Build history of the part. All positions in model axes, mm. Face numbers are marked on the shaded views. A direction names the side the tool comes from. Coordinates: 2 decimals unless noted, no trailing zeros. Order: outer loops, then holes, each group sorted by start corner. A loop starts at its lowest first (then second) coordinate and runs counter-clockwise, first axis right, second up. Notation, with made-up numbers: M 33.5,50 L 81.5,50 A22 cw 81.5,61 Z; hole C -27,50.5 d11. An arc over 180 degrees is marked long. Write item = value, one per line. Start each with the question number.
Q1. Band-saw the part on D-D on y = 1.3. Write the cut outline in (x, z), plus the area to 3 significant figures.
Q2. Pull direction X, two halves, no side cores. Call the marked faces 1, 2 and 3: released by +X, released by -X, zero draft, split by the parting line, or undercut.
Q3. Band-saw the part on C-C on y = 2.35. Write the cut outline in (x, z), plus the area to 3 significant figures.
Q4. Band-saw the part on B-B on z = 0. Write the cut outline in (x, y).
Q5. 3-axis set-ups, long thin cutter, end or side, ignore diameter. For the marked faces 4 and 5: which of +Z, -Z, +X, -X, +Y, -Y reach the whole face in a straight line?
Q6. Pin check, flat tips, straight feed: P1, Ø1.5, axis at x = -3.5, z = 1, coming from the -Y side; P2, Ø1.5, axis at y = 2.5, z = -2, coming from the +X side; P3, Ø1, axis at y = 3, z = 0, coming from the +X side. Stop position of each tip, or through.
Q7. Drill centre lines: probe 1 along X at (y, z) = (1.45, -0.25); probe 2 along X at (y, z) = (2.3, 0); probe 3 along Z at (x, y) = (1.75, 0.3). Where is each one in solid material? Low to high.
Q8. Band-saw the part on A-A on x = 0. Write the cut outline in (y, z), plus the area to 3 significant figures.
```python
from build123d import *

# Parameters (mm, degrees)
SKETCH2_R          = 0.5
CUT_EXTRUDE1_DEPTH = 8.329743599


with BuildPart() as part:
    # Sketch1 → Revolve1 (revolve)
    with BuildSketch(Plane.XY, mode=Mode.PRIVATE) as revolve1_sk:
        Polygon((0, 0), (3, 0), (2.5, 0.657540642), (3.702619215, 1.572023442), (3, 2.496024821), (4.5, 3.636638726), (0, 3.636638726), align=None)
    revolve(revolve1_sk.sketch.rotate(Axis((0, 3.636638726, 0), (0, -1, 0)), 90), axis=Axis((0, 3.636638726, 0), (0, -1, 0)))

    # Sketch2 → Cut-Extrude1 (cut, through all)
    with BuildSketch(Plane(origin=(0, 3.636638726, 0), x_dir=(1, 0, 0), z_dir=(0, 1, 0))):
        with Locations(Location((0, 0, 0), (0, 0, 270))):
            Circle(SKETCH2_R)
    extrude(amount=-CUT_EXTRUDE1_DEPTH, mode=Mode.SUBTRACT)


solid = part.part
```
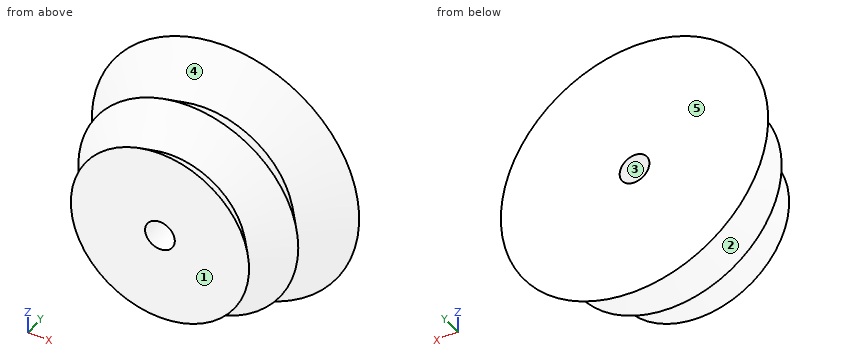
Recorded:
q1.outline = C 0,0 d6.69; hole C 0,0 d1
q1.area = 34.4 mm2
q2.face_1 = zero draft
q2.face_2 = split by the parting line
q2.face_3 = undercut
q3.outline = C 0,0 d6.22; hole C 0,0 d1
q3.area = 29.6 mm2
q4.outline = M -4.5,3.64 L -3,2.5 L -3.7,1.57 L -2.5,0.66 L -3,0 L -0.5,0 L -0.5,3.64 Z; M 0.5,0 L 3,0 L 2.5,0.66 L 3.7,1.57 L 3,2.5 L 4.5,3.64 L 0.5,3.64 Z
q5.face_4 = none
q5.face_5 = +Z, -Z, +X, -X, +Y
q6.P1 = 0
q6.P2 = 3.52
q6.P3 = 4.32
q7.probe_1 = -3.53 to -0.43, 0.43 to 3.53
q7.probe_2 = -3.15 to -0.5, 0.5 to 3.15
q7.probe_3 = -2.15 to 2.15
q8.outline = M 0,-3 L 0.66,-2.5 L 1.57,-3.7 L 2.5,-3 L 3.64,-4.5 L 3.64,-0.5 L 0,-0.5 Z; M 0,0.5 L 3.64,0.5 L 3.64,4.5 L 2.5,3 L 1.57,3.7 L 0.66,2.5 L 0,3 Z
q8.area = 20.4 mm2
